from build123d import *

# Parameters (mm, degrees)
PAD_DEPTH              = 6.25
FILLET_R               = 6.4
MIRROR_ROLL_ANGLE      = -179.860361
MIRROR_PITCH_ANGLE     = 0.86933
MIRROR_PLACEMENT_ANGLE = 0.335531


with BuildPart() as body:
    # Sketch → Pad (new body)
    with BuildSketch(Plane.XY):
        Polygon((0, 250), (50, 250), (150, 0), (120, 0), (120, 13.2), (30, 13.2), (30, 0), (0, 0), align=None)
        Polygon((15, 230), (15, 135), (79.844506, 135), (41.844506, 230), align=None, mode=Mode.SUBTRACT)
        Polygon((15, 115), (15, 33.2), (120.564506, 33.2), (87.844506, 115), align=None, mode=Mode.SUBTRACT)
        with BuildLine():
            ThreePointArc((18, 243.25), (14.75, 240), (18, 236.75))
            Line((18, 236.75), (38, 236.75))
            ThreePointArc((38, 236.75), (41.25, 240), (38, 243.25))
            Line((38, 243.25), (18, 243.25))
        make_face(mode=Mode.SUBTRACT)
        with BuildLine():
            ThreePointArc((60.5, 128.25), (57.25, 125), (60.5, 121.75))
            Line((60.5, 121.75), (80.5, 121.75))
            ThreePointArc((80.5, 121.75), (83.75, 125), (80.5, 128.25))
            Line((80.5, 128.25), (60.5, 128.25))
        make_face(mode=Mode.SUBTRACT)
        with BuildLine():
            ThreePointArc((18, 128.25), (14.75, 125), (18, 121.75))
            Line((18, 121.75), (38, 121.75))
            ThreePointArc((38, 121.75), (41.25, 125), (38, 128.25))
            Line((38, 128.25), (18, 128.25))
        make_face(mode=Mode.SUBTRACT)
        with BuildLine():
            ThreePointArc((18, 26.45), (14.75, 23.2), (18, 19.95))
            Line((18, 19.95), (38, 19.95))
            ThreePointArc((38, 19.95), (41.25, 23.2), (38, 26.45))
            Line((38, 26.45), (18, 26.45))
        make_face(mode=Mode.SUBTRACT)
        with BuildLine():
            ThreePointArc((101, 26.45), (97.75, 23.2), (101, 19.95))
            Line((101, 19.95), (121, 19.95))
            ThreePointArc((121, 19.95), (124.25, 23.2), (121, 26.45))
            Line((121, 26.45), (101, 26.45))
        make_face(mode=Mode.SUBTRACT)
    extrude(amount=PAD_DEPTH)

    # Fillet
    fillet_edges = [body.edges().sort_by_distance(p)[0] for p in [
        (0, 0, 3.125),
        (50, 250, 3.125),
        (0, 250, 3.125),
        (150, 0, 3.125),
        (120, 0, 3.125),
        (30, 0, 3.125),
        (41.844506, 230, 3.125),
        (15, 230, 3.125),
        (87.844506, 115, 3.125),
        (15, 115, 3.125),
        (15, 135, 3.125),
        (15, 33.2, 3.125),
        (120.564506, 33.2, 3.125),
        (79.844506, 135, 3.125),
        (30, 13.2, 3.125),
        (120, 13.2, 3.125),
    ]]
    fillet(fillet_edges, radius=FILLET_R)


with BuildPart() as body_mirrored:
    # mirror: instance of Body
    add(body.part.mirror(Plane(origin=(159.79538, 145.255219, 2.976273), x_dir=(0.000289, 1, 0), z_dir=(-1, 0.000289, -5.1e-05))))


with BuildPart() as body_mirrored_1:
    # mirror roll: moved
    add(body_mirrored.part.rotate(Axis((0, 0, 0), (1, 0, 0)), MIRROR_ROLL_ANGLE))


with BuildPart() as body_mirrored_2:
    # mirror pitch: moved
    add(body_mirrored_1.part.rotate(Axis((0, 0, 0), (0, 1, 0)), MIRROR_PITCH_ANGLE))


with BuildPart() as body_mirrored_3:
    # mirror placement: moved
    add(body_mirrored_2.part.moved(Location((-110.969424, 247.905415, 10.458181))).rotate(Axis((-110.969424, 247.905415, 10.458181), (0, 0, 1)), MIRROR_PLACEMENT_ANGLE))


solid = body_mirrored_3.part
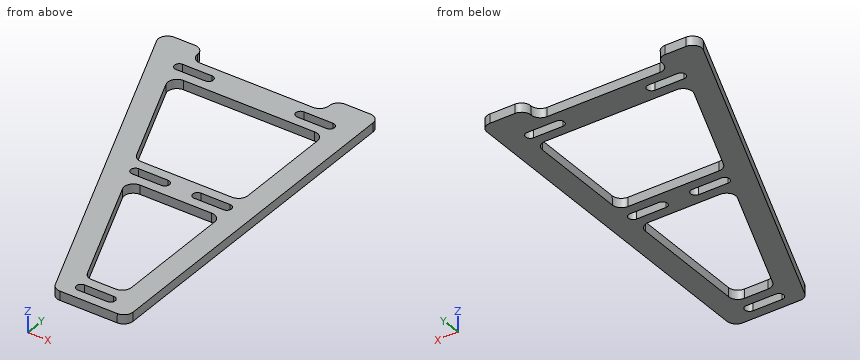
Can you work these out from the model? Positions are in its coordinate system, mm. Give positions to 0.01 mm unless a question says otherwise; leave off trailing zeros. Loops run counter-clockwise (first coordinate to the right, second up) from the corner with the lowest first, then second, coordinate; pieces in that order, holes last. Notation, with made-up numbers: M -4.75,6 L 6.25,6 A24 ccw 6.25,42 Z; hole C 43.25,88.5 d2. An arc over 180 degrees is marked long. One line per item, written item: value.
1) Imagine slicing it at B-B on x = 155. Write out the boundary of the cut face in (y, z), and give its area (3 significant figures).
Geometry check:
outline: M 11.85,-0.4 L 51.61,-0.3 L 51.83,5.95 L 12.07,5.85 Z; M 114.52,6.09 L 114.54,-0.16 L 134.54,-0.11 L 134.52,6.14 Z; M 216.32,6.33 L 216.34,0.08 L 236.34,0.13 L 236.32,6.38 Z
area: 499 mm²
2) Imagine slicing it at A-A on y = 159. Write out the boundary of the cut face in (x, z), and give its area (3 significant figures).
Geometry check:
outline: M 95.05,0.86 L 111.25,0.62 L 111.34,6.87 L 95.14,7.11 Z; M 193.98,-0.65 L 208.98,-0.88 L 209.08,5.37 L 194.08,5.6 Z
area: 195 mm²
3) Please list where these lines run through material, in increasing order: line 1 (Y direction, x = 134.5, z = 1); line 2 (Y direction, x = 158, z = 3); line 3 (Y direction, x = 143.5, z = 1.5).
Geometry check:
line 1: y = 62.21 to 101.96, 112.65 to 121.15, 127.65 to 134.4, 216.21 to 236.21
line 2: y = 4.61 to 44.36, 114.55 to 134.55, 216.35 to 236.35
line 3: y = 40.14 to 79.89, 114.46 to 121.21, 127.71 to 134.46, 216.26 to 236.26
4) Imagine slicing it at C-C on z = 3. Count the separate pieces of the cut face and the enclosed holes in it, and give its area (3 significant figures).
Geometry check:
separate pieces: 1
enclosed holes: 7
area: 11,400 mm²
5) I'm going to push flat-ended pins straight in: pin 1 (5 mm diameter, centred on x = 79, y = 214.5, fed in from -Z); pin 2 (1.5 mm diameter, centred on x = 117, z = 2.5, fed in from +Y); pin 3 (1 mm diameter, centred on x = 105, z = 4, fed in from +Y). Where does each tip first touch, or does it pass through?
Geometry check:
pin 1: stops at z = 1.2
pin 2: stops at y = 236.1
pin 3: stops at y = 236.01
